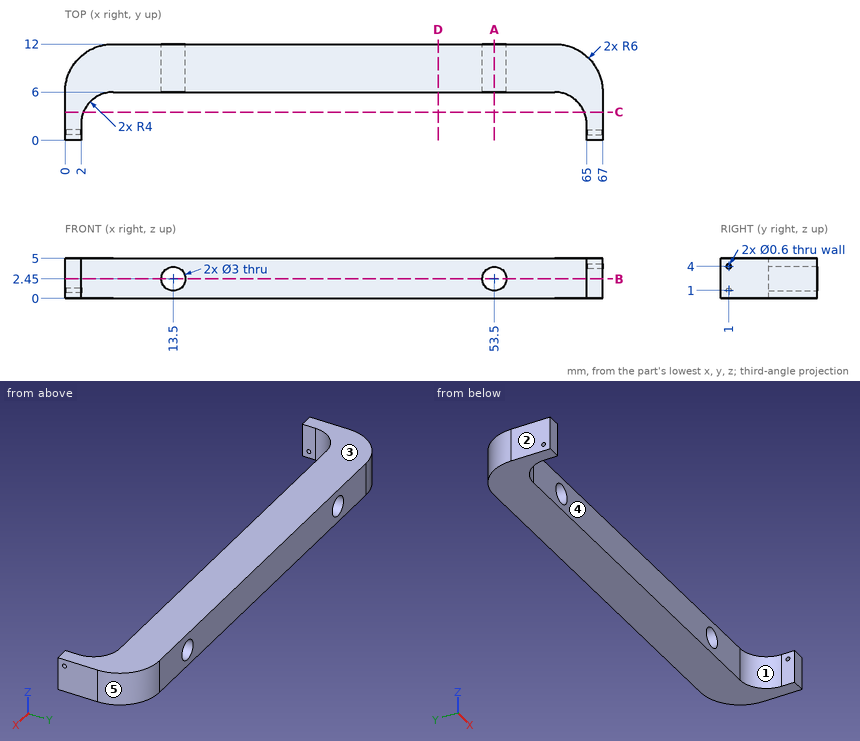
Here's the drawing with two shaded views (mm, measured from the low corner). I have some questions. A direction names the side the tool comes from. Coordinates: 2 decimals unless noted, no trailing zeros. Order: outer loops, then holes, each group sorted by start corner. A loop starts at its lowest first (then second) coordinate and runs counter-clockwise, first axis right, second up. Notation, with made-up numbers: (32.5, 25) - (43.5, 25) arc R30 ccw to (43.5, 64) - close; hole circle Ø2 at (46.25, 52). An arc over 180 degrees is marked (long way). Answer in a Markdown table with one row per item.
1. Suppose I cut it at A-A (x = 53.5). Please give me the cut outline in (y, z), and give its area (3 significant figures).
Reply:
| item | result |
|---|---|
| outline | (6, 0) - (12, 0) - (12, 0.95) - (6, 0.95) - close; (6, 3.95) - (12, 3.95) - (12, 5) - (6, 5) - close |
| area | 12.0 mm^2 |
2. Suppose I cut it at C-C (y = 3.5). Please give me the cut outline in (x, z), and give its area (3 significant figures).
Reply:
| item | result |
|---|---|
| outline | (0, 0) - (2.29, 0) - (2.29, 5) - (0, 5) - close; (64.71, 0) - (67, 0) - (67, 5) - (64.71, 5) - close |
| area | 22.9 mm^2 |
3. Suppose I cut it at D-D (x = 46.5). Please give me the cut outline in (y, z).
Reply:
| item | result |
|---|---|
| outline | (6, 0) - (12, 0) - (12, 5) - (6, 5) - close |
4. For the marked faces 1 and 2, which set-ups out of +Z, -Z, +X, -X, +Y, -Y let a thin tool reach every point of the face, with its end or its side?
Reply:
| item | result |
|---|---|
| face 1 | +Z, -Z, -Y |
| face 2 | +Z, -Z, -X, +Y, -Y |
5. Suppose I cut it at B-B (z = 2.45). Please give me the cut outline in (x, y), and give its area (3 significant figures).
Reply:
| item | result |
|---|---|
| outline | (0, 0) - (2, 0) - (2, 2) arc R4 cw to (6, 6) - (12, 6) - (12, 12) - (6, 12) arc R6 ccw to (0, 6) - close; (15, 6) - (52, 6) - (52, 12) - (15, 12) - close; (55, 6) - (61, 6) arc R4 cw to (65, 2) - (65, 0) - (67, 0) - (67, 6) arc R6 ccw to (61, 12) - (55, 12) - close |
| area | 381 mm^2 |
6. For pin 1 (4 mm diameter, centred on x = 20.5, y = 3, fed in from -Z), with a flat end and sliding along its axis, tell me the tip position at first contact or that it passes through.
Reply:
| item | result |
|---|---|
| pin 1 | passes through |
7. If I drill on line 1 along X through (y, z) = (0.5, 3.3); line 2 along X through (y, z) = (7.2, 2.45); line 3 along X through (y, z) = (7.75, 1.4), over which ranges is the centre line in solid material (lowest first)?
Reply:
| item | result |
|---|---|
| line 1 | x = 0 to 2, 65 to 67 |
| line 2 | x = 0.12 to 12, 15 to 52, 55 to 66.88 |
| line 3 | x = 0.26 to 12.43, 14.57 to 52.43, 54.57 to 66.74 |
8. If we mould it in two halves opening along X, with no side actions, what happens to the marked faces 3, 4 and 5? For each: pulls with the +X half, pulls with the -X half, needs draft (parallel to the pull), parting line crosses it, or undercut.
Reply:
| item | result |
|---|---|
| face 3 | needs draft |
| face 4 | undercut |
| face 5 | pulls with the +X half |
